Answer from the drawing. Dimensions are ordinates in mm from the lowest x, y and z of the part. A direction names the side the tool comes from. Coordinates: 2 decimals unless noted, no trailing zeros. Order: outer loops, then holes, each group sorted by start corner. A loop starts at its lowest first (then second) coordinate and runs counter-clockwise, first axis right, second up. Notation, with made-up numbers: M 80,-14.5 L 109,-14.5 A19 ccw 109,1.5 Z; hole C 47,38 d9. An arc over 180 degrees is marked long. Write each question's results on one line, items separated by ' | '.
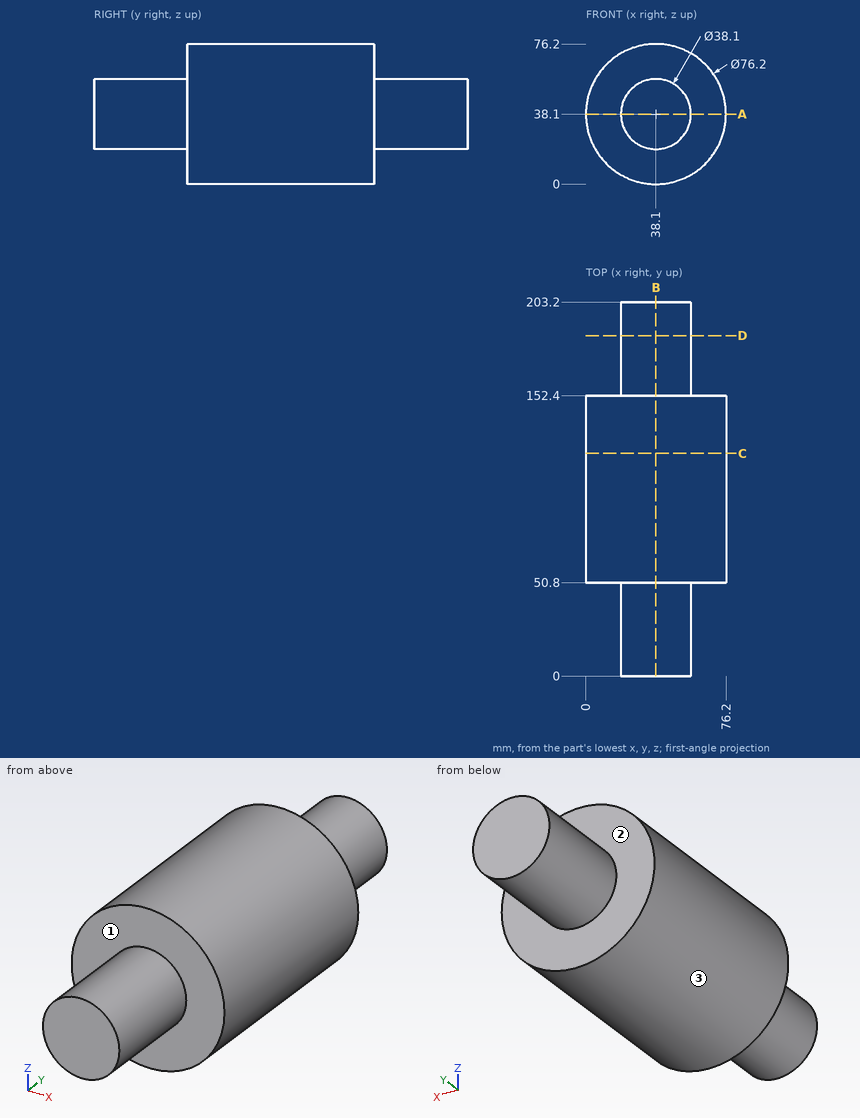
(1) For the marked faces 1, 2 and 3, determine the directions among +Z, -Z, +X, -X, +Y, -Y from which every point of the face is accessible in a straight line to the end or side of a thin tool.
Conclusion:
face 1: -Y | face 2: +Y | face 3: +Y, -Y
(2) The part is cut by section B-B, the plane x = 38.1. Write down the section's boundary in (y, z).
Conclusion:
outline: M 0,19.05 L 50.8,19.05 L 50.8,0 L 152.4,0 L 152.4,19.05 L 203.2,19.05 L 203.2,57.15 L 152.4,57.15 L 152.4,76.2 L 50.8,76.2 L 50.8,57.15 L 0,57.15 Z
(3) The part is cut by section C-C, the plane y = 121. Write down the section's boundary in (x, z).
Conclusion:
outline: C 38.1,38.1 d76.2
(4) The part is cut by section D-D, the plane y = 185. Write down the section's boundary in (x, z), then the cut area to 3 significant figures.
Conclusion:
outline: C 38.1,38.1 d38.1 | area: 1,140 mm²
(5) The part is cut by section A-A, the plane z = 38.1. Write down the section's boundary in (x, y), then the cut area to 3 significant figures.
Conclusion:
outline: M 0,50.8 L 19.05,50.8 L 19.05,0 L 57.15,0 L 57.15,50.8 L 76.2,50.8 L 76.2,152.4 L 57.15,152.4 L 57.15,203.2 L 19.05,203.2 L 19.05,152.4 L 0,152.4 Z | area: 11,600 mm²
(6) Given pin 1 (3 mm diameter, centred on x = 68.5, y = 78, fed in from -Z); pin 2 (2 mm diameter, centred on y = 65.5, z = 58, fed in from -X); pin 3 (4 mm diameter, centred on x = 11, z = 27.5, fed in from -Y), each flat-ended and moving along its own axis, determine where each tip first touches the part or whether it passes through.
Conclusion:
pin 1: z = 13.27 | pin 2: x = 5.02 | pin 3: y = 50.8
(7) Straight lines are drawn through the part: line 1 (Y direction, x = 65, z = 63); line 2 (Z direction, x = 37, y = 14); line 3 (Z direction, x = 39.5, y = 71.5). For each, find the intervals that lie inside material, in ascending order.
Conclusion:
line 1: 50.8 to 152.4 | line 2: 19.08 to 57.12 | line 3: 0.03 to 76.17
